from build123d import *

# Parameters (mm, degrees)
RESSALTO_EXTRUS_O1_DEPTH = 4
ESBO_O3_W                = 8.5
ESBO_O3_H                = 3
RESSALTO_EXTRUS_O2_DEPTH = 9.2
ESBO_O4_W                = 8.5
ESBO_O4_H                = 3
RESSALTO_EXTRUS_O3_DEPTH = 13
RESSALTO_EXTRUS_O6_DEPTH = 4
CORTE_EXTRUS_O3_DEPTH    = 7
ESBO_O9_W                = 5
ESBO_O9_H                = 4
RESSALTO_EXTRUS_O7_DEPTH = 1.5
ESBO_O10_R               = 2.75
CORTE_EXTRUS_O4_DEPTH    = 3


with BuildPart() as part:
    # Esboço1 → Ressalto-extrusão1 (new body)
    with BuildSketch(Plane.XY):
        Polygon((9.25, 0), (-9.25, 0), (-9.25, 3), (-4.25, 3), (-4.25, 6), (4.25, 6), (4.25, 3), (9.25, 3), align=None)
    extrude(amount=RESSALTO_EXTRUS_O1_DEPTH)

    # Esboço3 → Ressalto-extrusão2 (add)
    with BuildSketch(Plane.XY.offset(4)):
        with Locations((0, 4.5)):
            Rectangle(ESBO_O3_W, ESBO_O3_H)
    extrude(amount=RESSALTO_EXTRUS_O2_DEPTH)

    # Esboço4 → Ressalto-extrusão3 (add)
    with BuildSketch(Plane(origin=(4.25, 0, 0), x_dir=(0, 0, -1), z_dir=(1, 0, 0))):
        with Locations((-8.95, 4.5)):
            Rectangle(ESBO_O4_W, ESBO_O4_H)
    extrude(amount=RESSALTO_EXTRUS_O3_DEPTH)

    # Esboço5 → Ressalto-extrusão6 (add)
    with BuildSketch(Plane(origin=(17.25, 0, 0), x_dir=(0, 0, -1), z_dir=(1, 0, 0))):
        Polygon((-17.7, 0), (-17.7, 4.5), (-13.2, 4.5), (-13.2, 6), (-4.7, 6), (-4.7, 4.5), (-0.2, 4.5), (-0.2, 0), align=None)
    extrude(amount=RESSALTO_EXTRUS_O6_DEPTH)

    # Esboço8 → Corte-extrusão3 (cut, through all)
    with BuildSketch(Plane(origin=(0, 6, 0), x_dir=(1, 0, 0), z_dir=(0, 1, 0))):
        with BuildLine():
            Line((13.5, -6.2), (2.271563338, -6.2))
            ThreePointArc((2.271563338, -6.2), (-0.81107978, -5.122330007), (-2.75, -7.75))
            Line((-2.75, -7.75), (-2.75, -8.95))
            ThreePointArc((-2.75, -8.95), (-1.944543648, -10.894543648), (0, -11.7))
            Line((0, -11.7), (13.5, -11.7))
            ThreePointArc((13.5, -11.7), (16.25, -8.95), (13.5, -6.2))
        make_face()
    extrude(amount=-CORTE_EXTRUS_O3_DEPTH, mode=Mode.SUBTRACT)

    # Esboço9 → Ressalto-extrusão7 (add)
    with BuildSketch(Plane(origin=(0, 3, 0), x_dir=(1, 0, 0), z_dir=(0, 1, 0))):
        with Locations((-6.75, -2)):
            Rectangle(ESBO_O9_W, ESBO_O9_H)
        with Locations((6.75, -2)):
            Rectangle(ESBO_O9_W, ESBO_O9_H)
    extrude(amount=RESSALTO_EXTRUS_O7_DEPTH)

    # Esboço10 → Corte-extrusão4 (cut)
    with BuildSketch(Plane.XZ):
        with Locations((0, 5)):
            Circle(ESBO_O10_R)
        with Locations((16.25, 8.95)):
            Circle(ESBO_O10_R)
    extrude(amount=-CORTE_EXTRUS_O4_DEPTH, mode=Mode.SUBTRACT)


solid = part.part
Here's how the part is built. I have some questions about the finished solid (model axes, mm). A direction names the side the tool comes from. Coordinates: 2 decimals unless noted, no trailing zeros. Loops run counter-clockwise (first coordinate to the right, second up) from the corner with the lowest first, then second, coordinate; pieces in that order, holes last. Notation, with made-up numbers: (1, 86) -> (38, 86) arc R18 cw to (38, 114) -> close; hole circle Ø9 at (34, 71.25). An arc over 180 degrees is marked (long way). Use one line per item in the form item = value. Start each with the question number.
(1) If we section it at D-D (z = 9.5): Please give me the cut outline in (x, y), then the cut area to 4 significant figures.
(2) If we section it at C-C (y = 4.05): Please give me the cut outline in (x, z), then the cut area to 3 significant figures.
(3) Please list where these lines run through material, in increasing order: line 1 along Z through (x, y) = (7.5, 3.05); line 2 along X through (y, z) = (3.75, 2); line 3 along Z through (x, y) = (6, 5.4).
(4) Will these pins go through, and if not, where does the flat tip stop? pin 1 (1.5 mm diameter, centred on x = -6, y = 1.5, fed in from +Z); pin 2 (1.3 mm diameter, centred on y = 2.5, z = 13.5, fed in from -X); pin 3 (1.5 mm diameter, centred on x = -1, y = 4, fed in from +Z).
(5) If we section it at A-A (x = 12.5): Please give me the cut outline in (y, z), then the cut area to 3 significant figures.
(6) We'd pull the mould along X, two halves only. Please class faces 4 (the face through (-0.05, 1.48, 2.25)), 5 (the face through (19, 1, 9)), 6 (the face through (19, 4.5, 2)): pulls with the +X half, pulls with the -X half, needs draft (parallel to the pull), parting line crosses it, or undercut.
(7) On a 3-axis mill with a long thin cutter (end or side, diameter ignored), from which of +Z, -Z, +X, -X, +Y, -Y can I reach the whole of each face in a straight line? I mean faces 1 (the face through (-7, 4.5, 2)), 2 (the face through (19, 2, 0.2)), 3 (the face through (-1.97, 4.52, 10.87)). Say none if no direction works.
(8) If we section it at B-B (y = 0.7): Please give me the cut outline in (x, z), then the cut area to 3 significant figures.
Verdict:
q1.outline = (-4.25, 3) -> (-2.69, 3) -> (-2.69, 6) -> (-4.25, 6) -> close; (16.19, 3) -> (18.94, 3) -> (18.94, 0) -> (21.25, 0) -> (21.25, 6) -> (16.19, 6) -> close
q1.area = 26.75 mm²
q2.outline = (-9.25, 0) -> (9.25, 0) -> (9.25, 4) -> (4.25, 4) -> (4.25, 4.7) -> (17.25, 4.7) -> (17.25, 0.2) -> (21.25, 0.2) -> (21.25, 17.7) -> (17.25, 17.7) -> (17.25, 13.2) -> (-4.25, 13.2) -> (-4.25, 4) -> (-9.25, 4) -> close; hole (-2.75, 7.75) arc R2.75 ccw to (2.27, 6.2) -> (13.5, 6.2) arc R2.75 ccw to (13.5, 11.7) -> (0, 11.7) arc R2.75 ccw to (-2.75, 8.95) -> close
q2.area = 229 mm²
q3.line_1 = 0 to 4, 4.7 to 6.2, 11.7 to 13.2
q3.line_2 = -9.25 to 9.25, 17.25 to 21.25
q3.line_3 = 4.7 to 6.2, 11.7 to 13.2
q4.pin_1 = 4
q4.pin_2 = -4.25
q4.pin_3 = 13.2
q5.outline = (3, 4.7) -> (6, 4.7) -> (6, 6.2) -> (3, 6.2) -> close; (3, 11.7) -> (6, 11.7) -> (6, 13.2) -> (3, 13.2) -> close
q5.area = 9.00 mm²
q6.face_4 = undercut
q6.face_5 = pulls with the -X half
q6.face_6 = needs draft
q7.face_1 = +Z, -Z, -X, +Y
q7.face_2 = -Z, +X, +Y, -Y
q7.face_3 = +Y, -Y
q8.outline = (-9.25, 0) -> (9.25, 0) -> (9.25, 4) -> (2.56, 4) arc R2.75 cw to (-2.56, 4) -> (-9.25, 4) -> close; (17.25, 0.2) -> (21.25, 0.2) -> (21.25, 17.7) -> (17.25, 17.7) -> (17.25, 11.51) arc R2.75 cw to (17.25, 6.39) -> close
q8.area = 131 mm²
